from build123d import *

# Parameters (mm, degrees)
SKETCH2_W                                    = 100
SKETCH2_H                                    = 100
SKETCH2_W_2                                  = 50
SKETCH2_H_2                                  = 50
BOSS_EXTRUDE1_DEPTH                          = 10
CBORE_FOR_M6_HEX_SOCKET_HEAD_CAP_SCR_2_COUNT = 2
CBORE_FOR_M6_HEX_SOCKET_HEAD_CAP_SCR_2_PITCH = 75
CBORE_FOR_M6_HEX_SOCKET_HEAD_CAP_SCR_3_COUNT = 2
CBORE_FOR_M6_HEX_SOCKET_HEAD_CAP_SCR_3_PITCH = 106.066017178
CBORE_FOR_M6_HEX_SOCKET_HEAD_CAP_SCR_4_COUNT = 2
CBORE_FOR_M6_HEX_SOCKET_HEAD_CAP_SCR_4_PITCH = 75
SKETCH7_W                                    = 55
SKETCH7_H                                    = 55
SKETCH7_W_2                                  = 50
SKETCH7_H_2                                  = 50
BOSS_EXTRUDE2_DEPTH                          = 16
SKETCH8_W                                    = 11.008814293
SKETCH8_H                                    = 6
SKETCH8_R                                    = 2
SKETCH8_H_2                                  = 7.5
BOSS_EXTRUDE3_DEPTH                          = 5
SKETCH9_W                                    = 11.008814293
SKETCH9_H                                    = 7.5
SKETCH9_R                                    = 2
SKETCH9_H_2                                  = 6
CUT_EXTRUDE1_DEPTH                           = 1
FILLET1_R                                    = 3.2


with BuildPart() as part:
    # Sketch2 → Boss-Extrude1 (new body)
    with BuildSketch(Plane(origin=(0, 0, 0), x_dir=(0, 1, 0), z_dir=(0, 0, 1))):
        Rectangle(SKETCH2_W, SKETCH2_H)
        Rectangle(SKETCH2_W_2, SKETCH2_H_2, mode=Mode.SUBTRACT)
    extrude(amount=BOSS_EXTRUDE1_DEPTH)

    # Sketch6 → CBORE for M6 Hex Socket Head Cap Screw1 (revolve, cut)
    with BuildSketch(Plane(origin=(-37.5, 37.5, 10), x_dir=(0, -1, 0), z_dir=(1, 0, 0))):
        Polygon((0, 0), (0, 10), (3.3, 10), (3.3, 6.4), (5.5, 6.4), (5.5, 0.025), (5.525, 0), align=None)
    cbore_for_m6_hex_socket_head_cap_screw1 = revolve(axis=Axis((-37.5, 37.5, 16.35), (0, 0, -1)), mode=Mode.SUBTRACT)

    # CBORE for M6 Hex Socket Head Cap Scr 2: CBORE for M6 Hex Socket Head Cap Screw1 ×2
    with Locations(*[(i * CBORE_FOR_M6_HEX_SOCKET_HEAD_CAP_SCR_2_PITCH, 0, 0) for i in range(1, CBORE_FOR_M6_HEX_SOCKET_HEAD_CAP_SCR_2_COUNT)]):
        add(cbore_for_m6_hex_socket_head_cap_screw1, mode=Mode.SUBTRACT)

    # CBORE for M6 Hex Socket Head Cap Scr 3: CBORE for M6 Hex Socket Head Cap Screw1 ×2
    with Locations(*[Vector(0.7071067811865477, -0.7071067811865475, 0) * (i * CBORE_FOR_M6_HEX_SOCKET_HEAD_CAP_SCR_3_PITCH) for i in range(1, CBORE_FOR_M6_HEX_SOCKET_HEAD_CAP_SCR_3_COUNT)]):
        add(cbore_for_m6_hex_socket_head_cap_screw1, mode=Mode.SUBTRACT)

    # CBORE for M6 Hex Socket Head Cap Scr 4: CBORE for M6 Hex Socket Head Cap Screw1 ×2
    with Locations(*[(0, -i * CBORE_FOR_M6_HEX_SOCKET_HEAD_CAP_SCR_4_PITCH, 0) for i in range(1, CBORE_FOR_M6_HEX_SOCKET_HEAD_CAP_SCR_4_COUNT)]):
        add(cbore_for_m6_hex_socket_head_cap_screw1, mode=Mode.SUBTRACT)

    # Sketch7 → Boss-Extrude2 (add)
    with BuildSketch(Plane.XY.offset(10)):
        Rectangle(SKETCH7_W, SKETCH7_H)
        Rectangle(SKETCH7_W_2, SKETCH7_H_2, mode=Mode.SUBTRACT)
    extrude(amount=BOSS_EXTRUDE2_DEPTH)

    # Sketch8 → Boss-Extrude3 (add)
    # profile 1 of 4: a face of its own
    with BuildSketch(Plane.XY.offset(26)):
        with Locations((-19.495592853, 22)):
            Rectangle(SKETCH8_W, SKETCH8_H)
        with Locations((-20, 21.7015)):
            Circle(SKETCH8_R, mode=Mode.SUBTRACT)
    # profile 2 of 4: a face of its own
    with BuildSketch(Plane.XY.offset(26)):
        with Locations((19.495592853, 22)):
            Rectangle(SKETCH8_W, SKETCH8_H)
        with Locations((20, 21.7015)):
            Circle(SKETCH8_R, mode=Mode.SUBTRACT)
    # profile 3 of 4: a face of its own
    with BuildSketch(Plane.XY.offset(26)):
        with Locations((19.495592853, -21.25)):
            Rectangle(SKETCH8_W, SKETCH8_H_2)
        with Locations((20, -21.7015)):
            Circle(SKETCH8_R, mode=Mode.SUBTRACT)
    # profile 4 of 4: a face of its own
    with BuildSketch(Plane.XY.offset(26)):
        with Locations((-19.495592853, -21.25)):
            Rectangle(SKETCH8_W, SKETCH8_H_2)
        with Locations((-20, -21.7015)):
            Circle(SKETCH8_R, mode=Mode.SUBTRACT)
    extrude(amount=-BOSS_EXTRUDE3_DEPTH)

    # Sketch9 → Cut-Extrude1 (cut)
    # profile 1 of 4: a face of its own
    with BuildSketch(Plane.XY.offset(26)):
        with Locations((-19.495592853, -21.25)):
            Rectangle(SKETCH9_W, SKETCH9_H)
        with Locations((-20, -21.7015)):
            Circle(SKETCH9_R, mode=Mode.SUBTRACT)
    # profile 2 of 4: a face of its own
    with BuildSketch(Plane.XY.offset(26)):
        with Locations((19.495592853, -21.25)):
            Rectangle(SKETCH9_W, SKETCH9_H)
    # profile 3 of 4: a face of its own
    with BuildSketch(Plane.XY.offset(26)):
        with Locations((19.495592853, 22)):
            Rectangle(SKETCH9_W, SKETCH9_H_2)
    # profile 4 of 4: a face of its own
    with BuildSketch(Plane.XY.offset(26)):
        with Locations((-19.495592853, 22)):
            Rectangle(SKETCH9_W, SKETCH9_H_2)
    extrude(amount=-CUT_EXTRUDE1_DEPTH, mode=Mode.SUBTRACT)

    # Fillet1
    fillet1_edges = [part.edges().sort_by_distance(p)[0] for p in [
        (-13.991185707, -17.5, 23),
        (13.991185707, -17.5, 23),
        (13.991185707, 19, 23),
        (-13.991185707, 19, 23),
        (-27.5, -27.5, 18),
        (27.5, -27.5, 18),
        (27.5, 27.5, 18),
        (50, -50, 5),
        (-27.5, 27.5, 18),
        (-50, -50, 5),
        (-50, 50, 5),
        (50, 50, 5),
    ]]
    fillet(fillet1_edges, radius=FILLET1_R)


solid = part.part
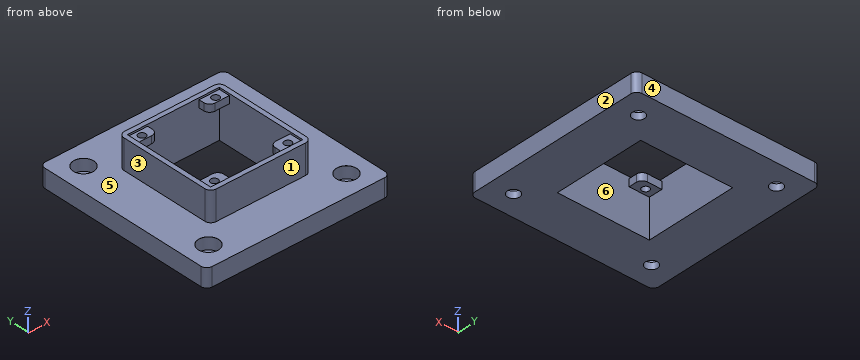
Check sheet for the modelled part. Datum: model origin and axes. Units: mm. Face numbers are marked on the shaded views. A direction names the side the tool comes from. Give positions to 0.01 mm unless a question says otherwise; leave off trailing zeros. Loops run counter-clockwise (first coordinate to the right, second up) from the corner with the lowest first, then second, coordinate; pieces in that order, holes last. Notation, with made-up numbers: M 17.5,78.5 L 32.5,78.5 A18 ccw 32.5,112.5 Z; hole C 11,58 d5. An arc over 180 degrees is marked long. Return JSON: item names as keys, results as strings. Group by question number.
1. Cross-section at A-A on x = -37.5. Record the boundary of the cut face in (y, z) (3 decimals).
2. Cross-section at B-B on y = -3.5. Record the boundary of the cut face in (x, z).
3. Cross-section at D-D on x = 20. Record the boundary of the cut face in (y, z).
4. Tool access check on the marked faces 1, 2 and 3. Record the directions out of +Z, -Z, +X, -X, +Y, -Y that give a thin tool (end or side, any length) a straight path to the whole face; none if there is none.
5. Cross-section at C-C on z = 5. Record the boundary of the cut face in (x, y), plus the area to 3 significant figures.
6. Go/stop test with flat-tipped pins: pin 1 (1.2 mm diameter, centred on x = -22, z = 23, fed in from +Y); pin 2 (8 mm diameter, centred on x = -20, y = -20, fed in from +Z); pin 3 (6 mm diameter, centred on x = -21.5, y = -21, fed in from -Z). Record where each tip stops, or that it passes through.
7. Mould release check, pull along Y, two halves, no side actions. Record for the marked faces 4, 5 and 6: released by +Y, released by -Y, zero draft, split by the parting line, or undercut.
8. Thickness scan on L1, parallel to X at y = -37.5, z = 2.65; L2, parallel to Y at x = 20, z = 22.75. Record the ranges inside material, lowest first.
Return value:
{
 "1": {"outline": "M -50,0 L -40.8,0 L -40.8,3.6 L -43,3.6 L -43,9.975 L -43.025,10 L -50,10 Z; M -34.2,0 L 34.2,0 L 34.2,3.6 L 32,3.6 L 32,9.975 L 31.975,10 L -31.975,10 L -32,9.975 L -32,3.6 L -34.2,3.6 Z; M 40.8,0 L 50,0 L 50,10 L 43.025,10 L 43,9.975 L 43,3.6 L 40.8,3.6 Z"},
 "2": {"outline": "M -50,0 L -25,0 L -25,26 L -27.5,26 L -27.5,10 L -50,10 Z; M 25,0 L 50,0 L 50,10 L 27.5,10 L 27.5,26 L 25,26 Z"},
 "3": {"outline": "M -50,0 L -25,0 L -25,21 L -23.7,21 L -23.7,25 L -25,25 L -25,26 L -27.5,26 L -27.5,10 L -50,10 Z; M -19.7,21 L -17.5,21 L -17.5,25 L -19.7,25 Z; M 19,21 L 19.7,21 L 19.7,25 L 19,25 Z; M 23.7,21 L 25,21 L 25,0 L 50,0 L 50,10 L 27.5,10 L 27.5,26 L 25,26 L 25,25 L 23.7,25 Z"},
 "4": {"face 1": "+Z, +X, -X, -Y", "face 2": "+Z, -Z, +X, +Y, -Y", "face 3": "+Z, -X, +Y, -Y"},
 "5": {"outline": "M -50,-46.8 A3.2 ccw -46.8,-50 L 46.8,-50 A3.2 ccw 50,-46.8 L 50,46.8 A3.2 ccw 46.8,50 L -46.8,50 A3.2 ccw -50,46.8 Z; hole C -37.5,-37.5 d11; hole C -37.5,37.5 d11; hole M -25,-25 L 25,-25 L 25,25 L -25,25 Z; hole C 37.5,-37.5 d11; hole C 37.5,37.5 d11", "area": "7,110 mm^2"},
 "6": {"pin 1": "y = 27.5", "pin 2": "z = 25", "pin 3": "z = 21"},
 "7": {"face 4": "released by +Y", "face 5": "zero draft", "face 6": "undercut"},
 "8": {"L1": "-50 to -40.8, -34.2 to 34.2, 40.8 to 50", "L2": "-27.5 to -23.7, -19.7 to -17.5, 19 to 19.7, 23.7 to 27.5"}
}
